from build123d import *

# Parameters (mm, degrees)
SKETCH1_W           = 139.7
SKETCH1_H           = 88.9
BOSS_EXTRUDE1_DEPTH = 19.05
SKETCH2_R           = 31.75
SKETCH2_R_2         = 19.05
BOSS_EXTRUDE2_DEPTH = 20.32
BOSS_EXTRUDE3_DEPTH = 12.7
SKETCH5_W           = 16.69963643
SKETCH5_H           = 76.2
BOSS_EXTRUDE4_DEPTH = 76.4794
CUT_EXTRUDE1_DEPTH  = 17.018


with BuildPart() as part:
    # Sketch1 → Boss-Extrude1 (new body)
    with BuildSketch(Plane(origin=(0, 0, 0), x_dir=(1, 0, 0), z_dir=(0, 1, 0))):
        Rectangle(SKETCH1_W, SKETCH1_H)
    extrude(amount=BOSS_EXTRUDE1_DEPTH)



with BuildPart() as body_2:
    # Sketch2 → Boss-Extrude2 (new body)
    with BuildSketch(Plane(origin=(0, 0, -44.45), x_dir=(-1, 0, 0), z_dir=(0, 0, -1))):
        with Locations((0, 127)):
            Circle(SKETCH2_R)
        with Locations((0, 127)):
            Circle(SKETCH2_R_2, mode=Mode.SUBTRACT)
    extrude(amount=-BOSS_EXTRUDE2_DEPTH)


with BuildPart() as part_1:
    add(part.part)

    add(body_2.part)  # Boss-Extrude3 merges body 2
    # Sketch3 → Boss-Extrude3 (add)
    with BuildSketch(Plane(origin=(0, 0, -44.45), x_dir=(-1, 0, 0), z_dir=(0, 0, -1))):
        with BuildLine():
            ThreePointArc((-31.75, 127), (0, 95.25), (31.75, 127))
            Line((31.75, 127), (69.85, 19.05))
            Line((69.85, 19.05), (-69.85, 19.05))
            Line((-69.85, 19.05), (-31.75, 127))
        make_face()
    extrude(amount=-BOSS_EXTRUDE3_DEPTH)

    # Sketch5 → Boss-Extrude4 (add)
    with BuildSketch(Plane(origin=(0, 19.05, 0), x_dir=(1, 0, 0), z_dir=(0, 1, 0))):
        with Locations((0, -6.35)):
            Rectangle(SKETCH5_W, SKETCH5_H)
    extrude(amount=BOSS_EXTRUDE4_DEPTH)

    # Sketch6 → Cut-Extrude1 (cut)
    with BuildSketch(Plane.ZY.offset(8.349818215)):
        Polygon((-24.13, 95.5294), (44.45, 19.05), (44.45, 95.5294), align=None)
    extrude(amount=-CUT_EXTRUDE1_DEPTH, mode=Mode.SUBTRACT)


solid = part_1.part
Read the model definition and answer for the solid it produces. Units are mm, in the model's axes. A direction names the side the tool comes from. Give positions to 0.01 mm unless a question says otherwise; leave off trailing zeros. Write each loop counter-clockwise with the first axis right and the second up, starting at its lowest first coordinate (ties: lowest second). Pieces come first, ordered by that corner, then holes. Notation, with made-up numbers: M 14.5,-2 L 34.5,-2 A23 ccw 34.5,15 Z; hole C -8.75,-17.75 d9. An arc over 180 degrees is marked long. One line per item, written item: value. Start each with the question number.
(1) Find section D-D (z = -6.5). Determine the outline of the cut face in (x, y), plus the area to 3 significant figures.
(2) Find section B-B (x = 0). Determine the outline of the cut face in (y, z).
(3) Find the intervals of material crossed by line 1 (Y direction, x = 0, z = -30.25); line 2 (Z direction, x = -39.5, y = 69.5); line 3 (Y direction, x = 13.5, z = 19.5), in increasing order.
(4) A tool of negligible diameter and unlimited length cuts with its end or side. For faces 1 (the flat face through (-69.85, 9, 1)), 2 (the flat face through (8.35, 48, -2)), 3 (the flat face through (-8.35, 48, -2)), from which of +Z, -Z, +X, -X, +Y, -Y can it reach the whole face along a straight path? Write none if from no direction.
(5) Determine the mould class of faces 4 (the cylindrical face through (-1.34, 158.72, -32.17)), 5 (the flat face through (-1, 0, -1)), 6 (the flat face through (-6, 95.529, -28)), 7 (the flat face through (-13.7, 113.5, -24.13)) for opening direction Y: pulls with the +Y half, pulls with the -Y half, needs draft (parallel to the pull), parting line crosses it, or undercut.
(6) Find section A-A (z = -37.5). Determine the outline of the cut face in (x, y), plus the area to 3 significant figures.
(7) Flat-ended cylindrical pins translate along their axes: pin 1 Ø1.2 at (x, z) = (-6, -30) entering from +Y; pin 2 Ø19.5 at (x, y) = (-23.5, 54.5) entering from +Z; pin 3 Ø3 at (y, z) = (66.5, -32.5) entering from -X. Find the tip coordinate at first contact, or state that the pin passes through.
(8) Find section C-C (y = 132). Determine the outline of the cut face in (x, z).
Results below:
1. outline: M -69.85,0 L 69.85,0 L 69.85,19.05 L 8.35,19.05 L 8.35,75.87 L -8.35,75.87 L -8.35,19.05 L -69.85,19.05 Z
1. area: 3,610 mm^2
2. outline: M 0,-44.45 L 107.95,-44.45 L 107.95,-24.13 L 95.53,-24.13 L 19.05,44.45 L 0,44.45 Z; M 146.05,-44.45 L 158.75,-44.45 L 158.75,-24.13 L 146.05,-24.13 Z
3. line 1: y = 0 to 107.95, 146.05 to 158.75
3. line 2: z = -44.45 to -31.75
3. line 3: y = 0 to 19.05
4. face 1: +Z, -Z, -X, +Y, -Y
4. face 2: +Z, +X
4. face 3: +Z, -X
5. face 4: undercut
5. face 5: pulls with the -Y half
5. face 6: undercut
5. face 7: needs draft
6. outline: M -69.85,0 L 69.85,0 L 69.85,19.05 L 31.75,127 A31.75 ccw -31.75,127 L -69.85,19.05 Z; hole C 0,127 d38.1
6. area: 14,100 mm^2
7. pin 1: stops at y = 158.29
7. pin 2: stops at z = -31.75
7. pin 3: stops at x = -53.63
8. outline: M -31.35,-44.45 L -18.38,-44.45 L -18.38,-24.13 L -31.35,-24.13 Z; M 18.38,-44.45 L 31.35,-44.45 L 31.35,-24.13 L 18.38,-24.13 Z
